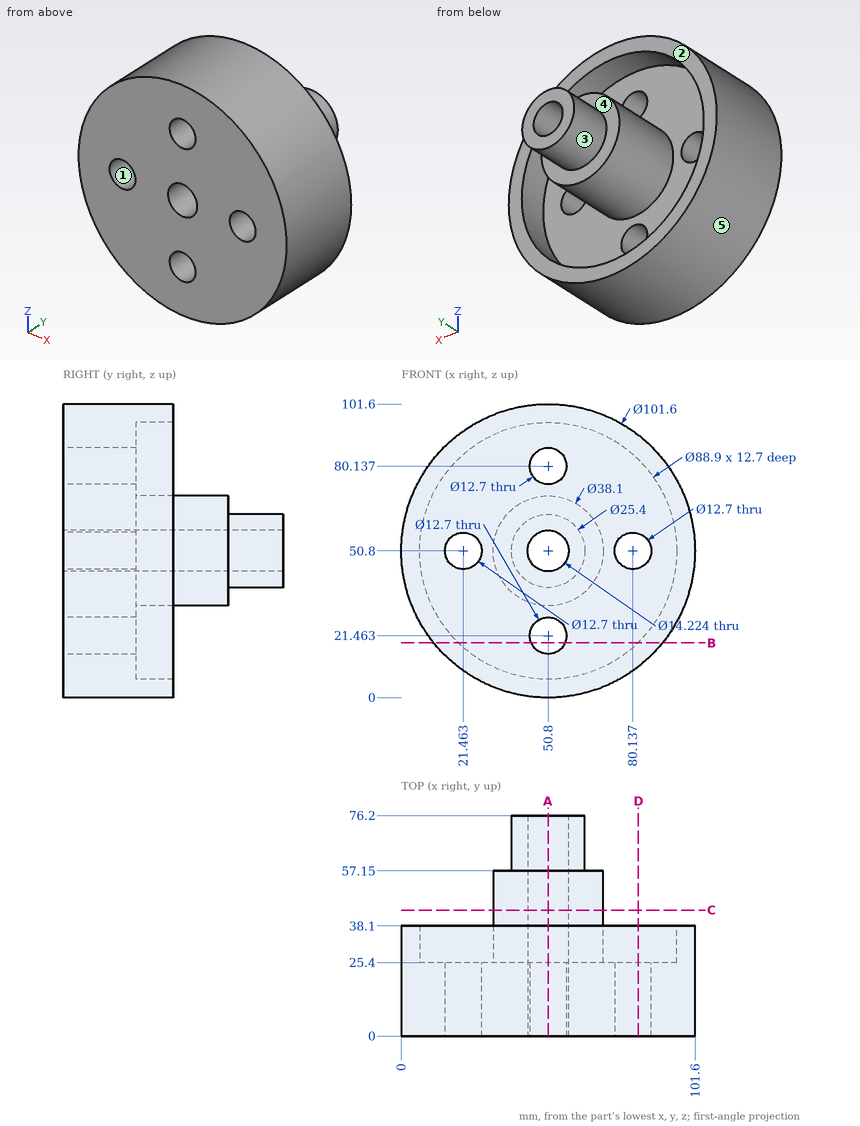
Verification items for this drawing (mm, ordinates from the low corner). A direction names the side the tool comes from. Coordinates: 2 decimals unless noted, no trailing zeros. Order: outer loops, then holes, each group sorted by start corner. A loop starts at its lowest first (then second) coordinate and runs counter-clockwise, first axis right, second up.
Q1. Sectioned sample at C-C on y = 43.5. Record the cut outline in (x, z), and give its area (3 significant figures).
Reply:
outline: circle Ø38.1 at (50.8, 50.8); hole circle Ø14.22 at (50.8, 50.8)
area: 981 mm2
Q2. Sectioned sample at D-D on x = 82. Record the cut outline in (y, z), and give its area (3 significant figures).
Reply:
outline: (0, 10.71) - (38.1, 10.71) - (38.1, 19.14) - (25.4, 19.14) - (25.4, 44.73) - (0, 44.73) - close; (0, 56.87) - (25.4, 56.87) - (25.4, 82.46) - (38.1, 82.46) - (38.1, 90.89) - (0, 90.89) - close
area: 1,940 mm2
Q3. Sectioned sample at B-B on z = 19. Record the cut outline in (x, y), and give its area (3 significant figures).
Reply:
outline: (11.18, 0) - (44.95, 0) - (44.95, 25.4) - (19.74, 25.4) - (19.74, 38.1) - (11.18, 38.1) - close; (56.65, 0) - (90.42, 0) - (90.42, 38.1) - (81.86, 38.1) - (81.86, 25.4) - (56.65, 25.4) - close
area: 1,930 mm2
Q4. Draft check along X on the marked faces 1, 2 and 3. Enter one of: released by +X, released by -X, zero draft, split by the parting line, or undercut.
Reply:
face 1: undercut
face 2: zero draft
face 3: split by the parting line
Q5. Sectioned sample at A-A on x = 50.8. Record the cut outline in (y, z), and give its area (3 significant figures).
Reply:
outline: (0, 0) - (38.1, 0) - (38.1, 6.35) - (25.4, 6.35) - (25.4, 15.11) - (0, 15.11) - close; (0, 27.81) - (25.4, 27.81) - (25.4, 31.75) - (57.15, 31.75) - (57.15, 38.1) - (76.2, 38.1) - (76.2, 43.69) - (0, 43.69) - close; (0, 57.91) - (76.2, 57.91) - (76.2, 63.5) - (57.15, 63.5) - (57.15, 69.85) - (25.4, 69.85) - (25.4, 73.79) - (0, 73.79) - close; (0, 86.49) - (25.4, 86.49) - (25.4, 95.25) - (38.1, 95.25) - (38.1, 101.6) - (0, 101.6) - close
area: 2,710 mm2
Q6. Tool access check on the marked faces 4 and 5. Record the directions out of +Z, -Z, +X, -X, +Y, -Y that give a thin tool (end or side, any length) a straight path to the whole face; none if there is none.
Reply:
face 4: +Y
face 5: +Y, -Y
Q7. Thickness scan on probe 1 along X at (y, z) = (29.75, 50.8); probe 2 along Z at (x, y) = (50.8, 14.75); probe 3 along Z at (x, y) = (47.5, 16). Record the ranges inside material, lowest first.
Reply:
probe 1: x = 0 to 6.35, 31.75 to 43.69, 57.91 to 69.85, 95.25 to 101.6
probe 2: z = 0 to 15.11, 27.81 to 43.69, 57.91 to 73.79, 86.49 to 101.6
probe 3: z = 0.11 to 16.04, 26.89 to 44.5, 57.1 to 74.71, 85.56 to 101.49
Q8. Depth check by flat-ended pin: pin 1 Ø1 at (y, z) = (11, 11.5) entering from -X; pin 2 Ø5 at (x, z) = (46, 69.5) entering from +Y; pin 3 Ø20.5 at (x, z) = (50.8, 80.137) entering from +Y. Enter the tip coordinate at first touch or a pass-through.
Reply:
pin 1: stops at x = 18.01
pin 2: stops at y = 57.15
pin 3: stops at y = 25.4
